Geometry check sheet. Reference: the model listing, model coordinates, mm. A direction names the side the tool comes from. Round coordinates to 2 decimals unless told otherwise and drop trailing zeros. Write each loop counter-clockwise with the first axis right and the second up, starting at its lowest first coordinate (ties: lowest second). Pieces come first, ordered by that corner, then holes. Notation, with made-up numbers: M 3.5,73 L 20.5,73 A15 ccw 20.5,92 Z; hole C 5.5,-32.5 d9. An arc over 180 degrees is marked long. Use a Markdown table: item, result.
```python
from build123d import *

# Parameters (mm, degrees)
SKETCH1_W            = 155
SKETCH1_H            = 5
BOSS_EXTRUDE2_DEPTH  = 55
SKETCH2_W            = 112
SKETCH2_H            = 45
SKETCH2_R            = 1.75
CUT_EXTRUDE1_DEPTH   = 55
SKETCH3_W            = 100
SKETCH3_H            = 20
CUT_EXTRUDE2_DEPTH   = 55
SKETCH4_W            = 40
SKETCH4_H            = 8.065867699
CUT_EXTRUDE3_DEPTH   = 55
BOSS_EXTRUDE4_DEPTH  = 5
CUT_EXTRUDE4_DEPTH   = 50
SKETCH9_W            = 4.377781836
SKETCH9_H            = 86.488706471
BOSS_EXTRUDE7_DEPTH  = 50
SKETCH10_W           = 20
SKETCH10_H           = 86.532324722
CUT_EXTRUDE5_DEPTH   = 10
SKETCH12_R           = 9.5
SKETCH12_R_2         = 6
CUT_EXTRUDE6_DEPTH   = 10
CUT_EXTRUDE7_START   = 50
SKETCH13_R           = 9.5
SKETCH13_R_2         = 6
CUT_EXTRUDE7_DEPTH   = 50
CUT_EXTRUDE8_DEPTH   = 50
CUT_EXTRUDE9_DEPTH   = 50
CUT_EXTRUDE10_DEPTH  = 10
FILLET5_R            = 3
SKETCH18_W           = 98.767816147
SKETCH18_H           = 10.604205858
BOSS_EXTRUDE8_DEPTH  = 5
CUT_EXTRUDE11_DEPTH  = 5
SKETCH20_W           = 155
SKETCH20_H           = 119
BOSS_EXTRUDE9_DEPTH  = 10
CUT_EXTRUDE13_DEPTH  = 155
SKETCH24_W           = 110
SKETCH24_H           = 8
BOSS_EXTRUDE10_DEPTH = 95
FILLET6_R            = 20
SKETCH26_W           = 16
SKETCH26_H           = 1.5
BOSS_EXTRUDE11_DEPTH = 12
BOSS_EXTRUDE12_DEPTH = 15
SKETCH28_R           = 2.5
CUT_EXTRUDE15_DEPTH  = 5
CUT_EXTRUDE17_DEPTH  = 35
SKETCH29_W           = 43
SKETCH29_H           = 43
CUT_EXTRUDE18_DEPTH  = 35
FILLET9_R            = 10
SKETCH31_W           = 124
SKETCH31_H           = 12
BOSS_EXTRUDE14_DEPTH = 2
SKETCH32_W           = 5
SKETCH32_H           = 2
BOSS_EXTRUDE15_DEPTH = 132
SKETCH33_W           = 20
SKETCH33_H           = 12
CUT_EXTRUDE19_DEPTH  = 160
SKETCH34_W           = 2
SKETCH34_H           = 12
BOSS_EXTRUDE17_DEPTH = 123
SKETCH36_R           = 6
CUT_EXTRUDE20_DEPTH  = 40
CUT_EXTRUDE21_DEPTH  = 25
SKETCH39_W           = 15
SKETCH39_H           = 12
CUT_EXTRUDE22_DEPTH  = 165
FILLET10_R           = 10
SKETCH40_W           = 2
SKETCH40_H           = 12
BOSS_EXTRUDE18_DEPTH = 115


with BuildPart() as part:
    # Sketch1 → Boss-Extrude2 (new body)
    with BuildSketch(Plane(origin=(0, 0, 0), x_dir=(1, 0, 0), z_dir=(0, 1, 0))):
        Polygon((-44.578450817, 29.59757322), (-48.782107146, 26.890310125), (-130, 153), (-125.796343671, 155.707263095), align=None)
        with BuildLine():
            ThreePointArc((0, 0), (-27.802696096, 7.256044178), (-48.782107146, 26.890310125))
            Line((-48.782107146, 26.890310125), (-44.578450817, 29.59757322))
            Line((-44.578450817, 29.59757322), (0, 5))
            Line((0, 5), (0, 0))
        make_face()
        with Locations((77.5, 2.5)):
            Rectangle(SKETCH1_W, SKETCH1_H)
    extrude(amount=BOSS_EXTRUDE2_DEPTH)

    # Sketch2 → Cut-Extrude1 (cut)
    with BuildSketch(Plane.XY):
        with Locations((99, 32.5)):
            Rectangle(SKETCH2_W, SKETCH2_H)
        with Locations((5, 25)):
            Circle(SKETCH2_R)
        with Locations((5, 50)):
            Circle(SKETCH2_R)
        with Locations((35, 50)):
            Circle(SKETCH2_R)
        with Locations((35, 25)):
            Circle(SKETCH2_R)
    extrude(amount=-CUT_EXTRUDE1_DEPTH, mode=Mode.SUBTRACT)

    # Sketch3 → Cut-Extrude2 (cut)
    with BuildSketch(Plane(origin=(-22.239707671, 0, 14.322945338), x_dir=(0.5414526190246729, 0, 0.840731265834287), z_dir=(-0.8407312658342869, 0, 0.5414526190246728))):
        with Locations((-99.020724146, 15)):
            Rectangle(SKETCH3_W, SKETCH3_H)
    extrude(amount=-CUT_EXTRUDE2_DEPTH, mode=Mode.SUBTRACT)

    # Sketch4 → Cut-Extrude3 (cut)
    with BuildSketch(Plane(origin=(2.114976352, 0, -3.832994761), x_dir=(-0.8755563671808256, 0, -0.48311597767939257), z_dir=(0.48311597767939257, 0, -0.8755563671808256))):
        with Locations((28.330006975, 9.03293385)):
            Rectangle(SKETCH4_W, SKETCH4_H)
    extrude(amount=-CUT_EXTRUDE3_DEPTH, mode=Mode.SUBTRACT)

    # Sketch5 → Boss-Extrude4 (add)
    with BuildSketch(Plane.XZ):
        Polygon((0, -5), (-44.578450817, -29.59757322), (-125.796343671, -155.707263095), (0, -155.707263095), align=None)
    extrude(amount=-BOSS_EXTRUDE4_DEPTH)

    # Sketch8 → Cut-Extrude4 (cut)
    with BuildSketch(Plane(origin=(0, 5, 0), x_dir=(1, 0, 0), z_dir=(0, 1, 0))):
        Polygon((-44.578450817, 29.59757322), (-98.72371272, 113.670699803), (-44.578450817, 113.670699803), align=None)
    extrude(amount=-CUT_EXTRUDE4_DEPTH, mode=Mode.SUBTRACT)

    # Sketch9 → Boss-Extrude7 (add)
    with BuildSketch(Plane(origin=(0, 5, 0), x_dir=(1, 0, 0), z_dir=(0, 1, 0))):
        with Locations((-42.389559899, 70.426346568)):
            Rectangle(SKETCH9_W, SKETCH9_H)
    extrude(amount=BOSS_EXTRUDE7_DEPTH)

    # Sketch10 → Cut-Extrude5 (cut)
    with BuildSketch(Plane(origin=(0, 5, 0), x_dir=(1, 0, 0), z_dir=(0, 1, 0))):
        with Locations((-30.200668981, 70.404537442)):
            Rectangle(SKETCH10_W, SKETCH10_H)
    extrude(amount=-CUT_EXTRUDE5_DEPTH, mode=Mode.SUBTRACT)

    # Sketch12 → Cut-Extrude6 (cut)
    with BuildSketch(Plane(origin=(-40.200668981, 0, 0), x_dir=(0, 0, -1), z_dir=(1, 0, 0))):
        with Locations(Location((57.181993332, 10, 0), (0, 0, 90))):
            Circle(SKETCH12_R)
        with Locations(Location((77.181993332, 10, 0), (0, 0, 90))):
            Circle(SKETCH12_R_2)
    extrude(amount=-CUT_EXTRUDE6_DEPTH, mode=Mode.SUBTRACT)

    # Sketch13 → Cut-Extrude7 (cut)
    with BuildSketch(Plane(origin=(-40.200668981, 0, 0), x_dir=(0, 0, -1), z_dir=(1, 0, 0)).offset(CUT_EXTRUDE7_START)):
        with Locations(Location((57.181993332, 10, 0), (0, 0, 90))):
            Circle(SKETCH13_R)
        with Locations(Location((77.181993332, 10, 0), (0, 0, 90))):
            Circle(SKETCH13_R_2)
    extrude(amount=-CUT_EXTRUDE7_DEPTH, mode=Mode.SUBTRACT)

    # Sketch14 → Cut-Extrude8 (cut)
    with BuildSketch(Plane(origin=(0, 5, 0), x_dir=(1, 0, 0), z_dir=(0, 1, 0))):
        Polygon((0, 103.038090201), (-91.876037903, 103.038090201), (-126.106254173, 155.707263095), (0, 155.707263095), align=None)
    extrude(amount=-CUT_EXTRUDE8_DEPTH, mode=Mode.SUBTRACT)

    # Sketch15 → Cut-Extrude9 (cut)
    with BuildSketch(Plane(origin=(-22.239707671, 0, 14.322945338), x_dir=(0.5414526190246729, 0, 0.840731265834287), z_dir=(-0.8407312658342869, 0, 0.5414526190246728))):
        Polygon((-176.035909688, 0), (-199.020724146, 18.247450711), (-199.020724146, 0), align=None)
    extrude(amount=-CUT_EXTRUDE9_DEPTH, mode=Mode.SUBTRACT)

    # Sketch16 → Cut-Extrude10 (cut)
    with BuildSketch(Plane(origin=(-40.200668981, 0, 0), x_dir=(0, 0, -1), z_dir=(1, 0, 0))):
        Polygon((113.670699803, 15.495236251), (48.252901996, 55), (113.670699803, 55), align=None)
    extrude(amount=-CUT_EXTRUDE10_DEPTH, mode=Mode.SUBTRACT)

    # Fillet5
    fillet5_edges = [part.edges().sort_by_distance(p)[0] for p in [
        (-100.847592598, 5, -112.302866383),
        (-46.680278982, 25, -28.243941672),
        (-46.680278982, 5, -28.243941672),
        (-100.825540884, 25, -112.317068256),
    ]]
    fillet(fillet5_edges, radius=FILLET5_R)

    # Sketch18 → Boss-Extrude8 (add)
    with BuildSketch(Plane(origin=(0, 5, 0), x_dir=(1, 0, 0), z_dir=(0, 1, 0))):
        with Locations((-49.383908074, 108.34019313)):
            Rectangle(SKETCH18_W, SKETCH18_H)
    extrude(amount=-BOSS_EXTRUDE8_DEPTH)

    # Sketch19 → Cut-Extrude11 (cut)
    with BuildSketch(Plane.XZ):
        Polygon((-97.82324149, -103.038090201), (-98.767816147, -104.504762295), (-98.767816147, -103.038090201), align=None)
    extrude(amount=-CUT_EXTRUDE11_DEPTH, mode=Mode.SUBTRACT)

    # Sketch20 → Boss-Extrude9 (add)
    with BuildSketch(Plane.XZ):
        with Locations((77.5, -64.5)):
            Rectangle(SKETCH20_W, SKETCH20_H)
    extrude(amount=-BOSS_EXTRUDE9_DEPTH)

    # Sketch21 → Cut-Extrude13 (cut)
    with BuildSketch(Plane(origin=(155, 0, 0), x_dir=(0, 0, -1), z_dir=(1, 0, 0))):
        Polygon((5, 10), (124, 10), (124, 7), align=None)
    extrude(amount=-CUT_EXTRUDE13_DEPTH, mode=Mode.SUBTRACT)

    # Sketch24 → Boss-Extrude10 (add)
    with BuildSketch(Plane.XZ):
        with Locations((70, -120)):
            Rectangle(SKETCH24_W, SKETCH24_H)
    extrude(amount=-BOSS_EXTRUDE10_DEPTH)

    # Fillet6
    fillet6_edges = [part.edges().sort_by_distance(p)[0] for p in [
        (70, 7.201680672, -116),
    ]]
    fillet(fillet6_edges, radius=FILLET6_R)

    # Sketch26 → Boss-Extrude11 (add)
    with BuildSketch(Plane(origin=(2.114976352, 0, -3.832994761), x_dir=(-0.8755563671808256, 0, -0.48311597767939257), z_dir=(0.48311597767939257, 0, -0.8755563671808256))):
        with Locations((28.330006975, 13.815867699)):
            Rectangle(SKETCH26_W, SKETCH26_H)
    extrude(amount=BOSS_EXTRUDE11_DEPTH)

    # Sketch27 → Boss-Extrude12 (add)
    with BuildSketch(Plane(origin=(0, 14.565867699, 0), x_dir=(1, 0, 0), z_dir=(0, 1, 0))):
        Polygon((-15.6850907, 13.654745957), (-9.887698968, 24.161422363), (-23.896600843, 31.891278006), (-29.693992575, 21.384601599), (-28.030435477, 20.466681242), (-23.150964103, 29.30980055), (-12.469176423, 23.415785623), (-17.348647798, 14.572666314), align=None)
    extrude(amount=BOSS_EXTRUDE12_DEPTH)

    # Sketch28 → Cut-Extrude15 (cut)
    with BuildSketch(Plane(origin=(0, 14.565867699, 0), x_dir=(1, 0, 0), z_dir=(0, 1, 0))):
        with Locations(Location((-20.24980595, 21.941233432, 0), (0, 0, 180))):
            Circle(SKETCH28_R)
    extrude(amount=-CUT_EXTRUDE15_DEPTH, mode=Mode.SUBTRACT)

    # Sketch25 → Cut-Extrude17 (cut)
    with BuildSketch(Plane(origin=(0, 0, -124), x_dir=(-1, 0, 0), z_dir=(0, 0, -1))):
        with BuildLine():
            Line((-36.75, 77), (-36.75, 72))
            ThreePointArc((-36.75, 72), (-35, 70.25), (-33.25, 72))
            Line((-33.25, 72), (-33.25, 77))
            ThreePointArc((-33.25, 77), (-35, 78.75), (-36.75, 77))
        make_face()
        with BuildLine():
            Line((-73.25, 77), (-73.25, 72))
            ThreePointArc((-73.25, 72), (-75, 70.25), (-76.75, 72))
            Line((-76.75, 72), (-76.75, 77))
            ThreePointArc((-76.75, 77), (-75, 78.75), (-73.25, 77))
        make_face()
    extrude(amount=-CUT_EXTRUDE17_DEPTH, mode=Mode.SUBTRACT)

    # Sketch29 → Cut-Extrude18 (cut)
    with BuildSketch(Plane.XY):
        with Locations((21.5, 33.5)):
            Rectangle(SKETCH29_W, SKETCH29_H)
    extrude(amount=-CUT_EXTRUDE18_DEPTH, mode=Mode.SUBTRACT)

    # Fillet9
    fillet9_edges = [part.edges().sort_by_distance(p)[0] for p in [
        (-115.522140631, 0, -134.985040643),
        (-127.898171835, 18.247450711, -154.353631548),
        (-42.389559899, 15.495236251, -113.670699803),
        (-42.389559899, 55, -48.252901996),
        (-127.898171835, 55, -154.353631548),
    ]]
    fillet(fillet9_edges, radius=FILLET9_R)

    # Sketch31 → Boss-Extrude14 (add)
    with BuildSketch(Plane(origin=(155, 0, 0), x_dir=(0, 0, -1), z_dir=(1, 0, 0))):
        with Locations((62, 6)):
            Rectangle(SKETCH31_W, SKETCH31_H)
    extrude(amount=-BOSS_EXTRUDE14_DEPTH)

    # Sketch32 → Boss-Extrude15 (add)
    with BuildSketch(Plane.ZY.offset(-153)):
        with Locations((-2.5, 11)):
            Rectangle(SKETCH32_W, SKETCH32_H)
    extrude(amount=BOSS_EXTRUDE15_DEPTH)

    # Sketch33 → Cut-Extrude19 (cut)
    with BuildSketch(Plane.XY):
        with Locations((145, 6)):
            Rectangle(SKETCH33_W, SKETCH33_H)
    extrude(amount=-CUT_EXTRUDE19_DEPTH, mode=Mode.SUBTRACT)

    # Sketch34 → Boss-Extrude17 (add)
    with BuildSketch(Plane.XY):
        with Locations((134, 6)):
            Rectangle(SKETCH34_W, SKETCH34_H)
    extrude(amount=-BOSS_EXTRUDE17_DEPTH)

    # Sketch36 → Cut-Extrude20 (cut, symmetric)
    with BuildSketch(Plane(origin=(-40.200668981, 0, 0), x_dir=(0, 0, -1), z_dir=(1, 0, 0))):
        with Locations(Location((90.194878088, 10, 0), (0, 0, 90))):
            Circle(SKETCH36_R)
    extrude(amount=CUT_EXTRUDE20_DEPTH, both=True, mode=Mode.SUBTRACT)

    # Sketch38 → Cut-Extrude21 (cut)
    with BuildSketch(Plane(origin=(125, 0, 0), x_dir=(0, 0, -1), z_dir=(1, 0, 0))):
        Polygon((95.495958465, 7.718589282), (124, 7), (124, 95), (116, 95), align=None)
    extrude(amount=-CUT_EXTRUDE21_DEPTH, mode=Mode.SUBTRACT)

    # Sketch39 → Cut-Extrude22 (cut)
    with BuildSketch(Plane.XY):
        with Locations((127.5, 6)):
            Rectangle(SKETCH39_W, SKETCH39_H)
    extrude(amount=-CUT_EXTRUDE22_DEPTH, mode=Mode.SUBTRACT)

    # Fillet10
    fillet10_edges = [part.edges().sort_by_distance(p)[0] for p in [
        (0, 12, -2.5),
        (0, 55, -2.5),
    ]]
    fillet(fillet10_edges, radius=FILLET10_R)

    # Sketch40 → Boss-Extrude18 (add)
    with BuildSketch(Plane.XY):
        with Locations((119, 6)):
            Rectangle(SKETCH40_W, SKETCH40_H)
    extrude(amount=-BOSS_EXTRUDE18_DEPTH)


solid = part.part
```
Item 1: Cross-section at C-C, the plane x = 22. Record the cut outline in (y, z).
Outcome:
| item | result |
|---|---|
| outline | M 0,-124 L 95,-124 L 95,-116 L 27.71,-116 A20 cw 7.72,-95.5 L 10,-5 L 12,-5 L 12,0 L 0,0 Z |
Item 2: Cross-section at D-D, the plane y = 88.5. Record the cut outline in (x, z).
Outcome:
| item | result |
|---|---|
| outline | M 15,-124 L 100,-124 L 100,-116 L 15,-116 Z |
Item 3: Material ranges on line 1 along Z through (x, y) = (-43, 10); line 2 along Z through (x, y) = (-41, 10); line 3 along Z through (x, y) = (45, 74), recorded low to high. Write a range as from..to.
Outcome:
| item | result |
|---|---|
| line 1 | z = -113.67..-96.19, -84.19..-83.18, -71.18..-66.68, -47.68..-22.11 |
| line 2 | z = -113.67..-96.19, -84.19..-83.18, -71.18..-66.68, -47.68..-25.73 |
| line 3 | z = -124..-116 |
Item 4: Mould release check, pull along Y, two halves, no side actions. Record for faces 1 (the face through (-42.36, 8.7, -83.04)), 2 (the face through (-121.358, 8.615, -144.134)), 3 (the face through (-14.875, 21.961, -19.056)), 4 (the face through (118.2, 12, -32.2)): +Y half, -Y half, draft (parallel to the pull), parting line (faces both ways), or undercut.
Outcome:
| item | result |
|---|---|
| face 1 | undercut |
| face 2 | -Y half |
| face 3 | draft |
| face 4 | +Y half |
Item 5: Cross-section at B-B, the plane x = -82.5. Record the cut outline in (y, z), and give its area (3 significant figures).
Outcome:
| item | result |
|---|---|
| outline | M 0,-113.64 L 5,-113.64 L 5,-103.04 L 0,-103.04 Z; M 0,-88.48 L 5,-88.48 L 5,-79.25 L 0,-79.25 Z; M 25,-88.48 L 55,-88.48 L 55,-79.25 L 25,-79.25 Z |
| area | 376 mm2 |
Item 6: Access from +Z, -Z, +X, -X, +Y, -Y to the whole of each face (thin tool, end or side, straight path). Record for faces 5 (the face through (-17.88, 21.96, -26.4)), 6 (the face through (-100.333, 24.098, -111.617)), 7 (the face through (15, 48, -119)), 8 (the face through (-42.36, 35.74, -80.15)).
Outcome:
| item | result |
|---|---|
| face 5 | +Y |
| face 6 | +Z, +X |
| face 7 | -Z, +Y |
| face 8 | -Z, +X, +Y |
Item 7: Go/stop test with flat-tipped pins: pin 1 (8 mm diameter, centred on x = -20.25, z = -21.94, fed in from +Y); pin 2 (5 mm diameter, centred on x = -43, y = 8.5, fed in from -Z); pin 3 (22 mm diameter, centred on y = 10, z = -57.18, fed in from -X). Record where each tip stops, or that it passes through.
Outcome:
| item | result |
|---|---|
| pin 1 | stops at y = 14.57 |
| pin 2 | stops at z = -113.67 |
| pin 3 | stops at x = -74.6 |
Item 8: Cross-section at A-A, the plane y = 41. Record the cut outline in (x, z), and give its area (3 significant figures).
Outcome:
| item | result |
|---|---|
| outline | M -130,-153 L -125.8,-155.71 L -44.58,-29.6 L -44.58,-71.44 L -40.2,-71.44 L -40.2,-27.18 L 0,-5 L 0,0 A58.41 ccw -48.78,-26.89 Z; M 15,-124 L 100,-124 L 100,-116 L 15,-116 Z |
| area | 2,120 mm2 |
